Check sheet for the modelled part. Datum: model origin and axes. Units: mm. A direction names the side the tool comes from. Give positions to 0.01 mm unless a question says otherwise; leave off trailing zeros. Order: outer loops, then holes, each group sorted by start corner. A loop starts at its lowest first (then second) coordinate and runs counter-clockwise, first axis right, second up. Notation, with made-up numbers: (-14.75, 75) -> (15.25, 75) arc R21 ccw to (15.25, 99) -> close; hole circle Ø4 at (86, 6.25). An arc over 180 degrees is marked (long way). Write each question's results on one line, items separated by ' | '.
from build123d import *

# Parameters (mm, degrees)
SKETCH022_R     = 1.75
SKETCH022_R_2   = 2.25
PAD009_DEPTH    = 3
POCKET019_DEPTH = 1.5
PAD014_DEPTH    = 2


with BuildPart() as part:
    # Sketch022 → Pad009 (new body)
    with BuildSketch(Plane.XZ):
        Polygon((30.5, 48), (2.5, 48), (2.5, 31.5), (16, -10), (16, -30), (30.5, -30), align=None)
        with Locations((19.5, -24)):
            Circle(SKETCH022_R, mode=Mode.SUBTRACT)
        with Locations((9.5, 31.5)):
            Circle(SKETCH022_R_2, mode=Mode.SUBTRACT)
        with Locations((26.5, 35)):
            Circle(SKETCH022_R, mode=Mode.SUBTRACT)
    extrude(amount=-PAD009_DEPTH)

    # Sketch036 → Pocket019 (cut)
    with BuildSketch(Plane.XZ):
        Polygon((12.3145825623, 29.875), (12.3145825623, 33.125), (9.5, 34.75), (6.6854174377, 33.125), (6.6854174377, 29.875), (9.5, 28.25), align=None)
    extrude(amount=-POCKET019_DEPTH, mode=Mode.SUBTRACT)

    # Sketch039 → Pad014 (join)
    with BuildSketch(Plane.XZ):
        Polygon((22.25, 36.75), (22.25, 22.75), (27.25, 22.75), (27.25, 19.75), (19.25, 19.75), (19.25, 36.75), align=None)
    extrude(amount=PAD014_DEPTH)


with BuildPart() as part_1:
    # Body004 placement: moved
    add(part.part.moved(Location((0, 40, 0))))


solid = part_1.part
1. Section check B-B on y = 42.3. Record the cut outline in (x, z), then the cut area to 3 significant figures.
Verdict:
outline: (2.5, 31.5) -> (16, -10) -> (16, -30) -> (30.5, -30) -> (30.5, 48) -> (2.5, 48) -> close; hole circle Ø4.5 at (9.5, 31.5); hole circle Ø3.5 at (19.5, -24); hole circle Ø3.5 at (26.5, 35) | area: 1,600 mm^2
2. Access from +Z, -Z, +X, -X, +Y, -Y to the whole of each face (thin tool, end or side, straight path). Record for faces 1 (the flat face through (7, 41.5, 32)), 2 (the flat face through (22.25, 39, 30)), 3 (the flat face through (27.25, 39, 21)), 4 (the flat face through (23, 39, 19.75)), 5 (the flat face through (21, 39, 36.75)).
Verdict:
face 1: -Y | face 2: +Z, +X, -Y | face 3: +Z, -Z, +X, -Y | face 4: -Z, +X, -X, -Y | face 5: +Z, +X, -X, -Y
3. Section check A-A on x = 26.5. Record the cut outline in (y, z).
Verdict:
outline: (38, 19.75) -> (40, 19.75) -> (40, -30) -> (43, -30) -> (43, 33.25) -> (40, 33.25) -> (40, 22.75) -> (38, 22.75) -> close; (40, 36.75) -> (43, 36.75) -> (43, 48) -> (40, 48) -> close
4. Section check C-C on z = -16.5. Record the cut outline in (x, y).
Verdict:
outline: (16, 40) -> (30.5, 40) -> (30.5, 43) -> (16, 43) -> close
5. Section check D-D on y = 39.05. Record the cut outline in (x, z), then the cut area to 3 significant figures.
Verdict:
outline: (19.25, 19.75) -> (27.25, 19.75) -> (27.25, 22.75) -> (22.25, 22.75) -> (22.25, 36.75) -> (19.25, 36.75) -> close | area: 66.0 mm^2
6. Mould release check, pull along X, two halves, no side actions. Record for faces 6 (the flat face through (19, 40, 18)), 7 (the cylindrical face through (19.272, 41.479, -22.265)), 8 (the flat face through (19.25, 39, 28)): +X half, -X half, draft (parallel to the pull), parting line (faces both ways), or undercut.
Verdict:
face 6: draft | face 7: undercut | face 8: -X half
7. Material ranges on probe 1 along Z at (x, y) = (19.5, 40.7); probe 2 along Z at (x, y) = (26.5, 41.9); probe 3 along Y at (x, z) = (11.5, 8.5), recorded low to high. Write a range as from..to.
Verdict:
probe 1: z = -30..-25.75, -22.25..48 | probe 2: z = -30..33.25, 36.75..48 | probe 3: y = 40..43
8. Gauge pin test, flat ends, axial feed: pin 1 Ø0.6 at (y, z) = (39.5, 21) entering from +X; pin 2 Ø0.6 at (x, y) = (26, 39) entering from +Z; pin 3 Ø4 at (x, z) = (19.5, -24) entering from -Y. Record the tip position at first contact, or that the pin passes through.
Verdict:
pin 1: stops at x = 27.25 | pin 2: stops at z = 22.75 | pin 3: stops at y = 40
